Autodesk Inventor part; units mm, degrees
ref_plane "YZ Plane" through (0, 0, 0) normal (1, 0, 0) x (0, 1, 0)
ref_plane "XZ Plane" through (0, 0, 0) normal (0, 1, 0) x (-1, 0, 0)
ref_plane "XY Plane" through (0, 0, 0) normal (0, 0, 1) x (1, 0, 0)
sketch "Sketch1" plane through (0, 0, 0) normal (0, 1, 0) x (-1, 0, 0)
  circle A0 centre (0, 0) radius 18
  dimension "d0" = 36
extrude "Extrusion1" add sketch "Sketch1" along normal blind 100
sketch "Sketch3" plane through (0, 100, 0) normal (0, 1, 0) x (1, 0, 0)
  circle A0 centre (0, 0) radius 18
  line L0 (-10, 14.9666) -> (10, 14.9666)
  circle A1 centre (0, 0) radius 18
  line L1 (0, 0) -> (10, 0)
  line L2 (-10, -14.9666) -> (10, -14.9666)
  point P0 (0, 14.9666)
  point P1 (10, 14.9666)
  point P2 (10, -14.9666)
  dimension "d6" = 20
extrude "Extrusion3" cut sketch "Sketch3" against normal blind 10 contours L0 A0 | A0 L2
sketch "Sketch4" plane through (10, 100, -14.9666) normal (0, 0, -1) x (-1, 0, 0)
  arc A0 (6.5, -7) -> (3.5, -7) centre (5, -5) ccw
  arc A1 (16.5, -7) -> (13.5, -7) centre (15, -5) ccw
  circle A2 centre (5, -5) radius 2.5
  circle A3 centre (15, -5) radius 2.5
  point P0 (10, -100)
  point P1 (3.5, -7)
  point P2 (6.5, -7)
  point P3 (13.5, -7)
  point P4 (16.5, -7)
extrude "Extrusion4" cut sketch "Sketch4" against normal through all
sketch "Sketch5" plane through (0, 0, 0) normal (0, -1, 0) x (1, 0, 0)
  circle A0 centre (13.5, 0) radius 1.5
  circle A1 centre (0, 13.5) radius 1.5
  circle A2 centre (-13.5, 0) radius 1.5
  circle A3 centre (0, -13.5) radius 1.5
  point P0 (0, 0)
  dimension "d11" = 3
  dimension "d12" = 13.5
  dimension "d15" = 360
extrude "Extrusion5" cut sketch "Sketch5" against normal blind 8
properties part number "link1"
Check sheet for the modelled part. Datum: model origin and axes. Units: mm. A direction names the side the tool comes from. Give positions to 0.01 mm unless a question says otherwise; leave off trailing zeros. Write each loop counter-clockwise with the first axis right and the second up, starting at its lowest first coordinate (ties: lowest second). Pieces come first, ordered by that corner, then holes. Notation, with made-up numbers: (7.25, 21) -> (42.25, 21) arc R17 cw to (42.25, 31) -> close; hole circle Ø5 at (55.5, -31). An arc over 180 degrees is marked (long way). One line per item, written item: value. Start each with the question number.
Item 1: Section check A-A on z = 0. Record the cut outline in (x, y), then the cut area to 3 significant figures.
Item 2: Section check C-C on x = -5. Record the cut outline in (y, z), then the cut area to 3 significant figures.
Item 3: Tool access check on faces 1 (the flat face through (0, 95, -14.967)), 2 (the flat face through (-14, 8, 0)), 3 (the flat face through (0, 95, 14.967)). Record the directions out of +Z, -Z, +X, -X, +Y, -Y that give a thin tool (end or side, any length) a straight path to the whole face; none if there is none.
Item 4: Gauge pin test, flat ends, axial feed: pin 1 (4 mm diameter, centred on x = -5, y = 95, fed in from +Z); pin 2 (4 mm diameter, centred on y = 40, z = -6, fed in from +X); pin 3 (1.5 mm diameter, centred on x = -10.5, y = 49.5, fed in from -Z); pin 4 (5 mm diameter, centred on x = -5, y = 97.5, fed in from -Z). Record the tip position at first contact, or that the pin passes through.
Item 5: Material ranges on probe 1 along Z at (x, y) = (0, 3.5); probe 2 along Y at (x, z) = (5, -5.25); probe 3 along X at (y, z) = (95, 2.5), recorded low to high. Write a range as from..to.
Item 6: Section check D-D on x = 0. Record the cut outline in (y, z).
Item 7: Section check B-B on y = 95. Record the cut outline in (x, z).
Item 8: Draft check along X on faces 4 (the cylindrical face through (0, 4, 12)), 5 (the cylindrical face through (-5.62, 92.58, -0.21)), 6 (the flat face through (0, 100, 0)), 7 (the cylindrical face through (17.983, 49.3, -0.791)). Enter one of: +X half, -X half, draft (parallel to the pull), parting line (faces both ways), or undercut.
Results list:
1. outline: (-18, 0) -> (-15, 0) -> (-15, 8) -> (-12, 8) -> (-12, 0) -> (12, 0) -> (12, 8) -> (15, 8) -> (15, 0) -> (18, 0) -> (18, 100) -> (-18, 100) -> close; hole circle Ø5 at (-5, 95); hole circle Ø5 at (5, 95)
1. area: 3,510 mm²
2. outline: (0, -17.29) -> (90, -17.29) -> (90, -14.97) -> (92.5, -14.97) -> (92.5, 14.97) -> (90, 14.97) -> (90, 17.29) -> (0, 17.29) -> close; (97.5, -14.97) -> (100, -14.97) -> (100, 14.97) -> (97.5, 14.97) -> close
2. area: 3,260 mm²
3. face 1: -Z, +X, -X, +Y
3. face 2: -Y
3. face 3: +Z, +X, -X, +Y
4. pin 1: through
4. pin 2: x = 17.55
4. pin 3: z = -15.13
4. pin 4: z = -14.97
5. probe 1: -18..-15, -12..12, 15..18
5. probe 2: 0..92.5, 97.5..100
5. probe 3: -17.83..-7.5, -2.5..2.5, 7.5..17.83
6. outline: (0, -18) -> (90, -18) -> (90, -14.97) -> (100, -14.97) -> (100, 14.97) -> (90, 14.97) -> (90, 18) -> (0, 18) -> (0, 15) -> (8, 15) -> (8, 12) -> (0, 12) -> (0, -12) -> (8, -12) -> (8, -15) -> (0, -15) -> close
7. outline: (-10, -14.97) -> (-7.5, -14.97) -> (-7.5, 14.97) -> (-10, 14.97) arc R18 ccw to start; (-2.5, -14.97) -> (2.5, -14.97) -> (2.5, 14.97) -> (-2.5, 14.97) -> close; (7.5, -14.97) -> (10, -14.97) arc R18 ccw to (10, 14.97) -> (7.5, 14.97) -> close
8. face 4: undercut
8. face 5: undercut
8. face 6: draft
8. face 7: parting line
